Design review of the part built by this model. Coordinates are the model's own, in mm. Face numbers are marked on the shaded views. A direction names the side the tool comes from. Give positions to 0.01 mm unless a question says otherwise; leave off trailing zeros. Loops run counter-clockwise (first coordinate to the right, second up) from the corner with the lowest first, then second, coordinate; pieces in that order, holes last. Notation, with made-up numbers: (50, -19.5) - (77, -19.5) arc R35 ccw to (77, 12.5) - close; hole circle Ø9 at (45.5, -14). An arc over 180 degrees is marked (long way). One line per item, written item: value. Start each with the question number.
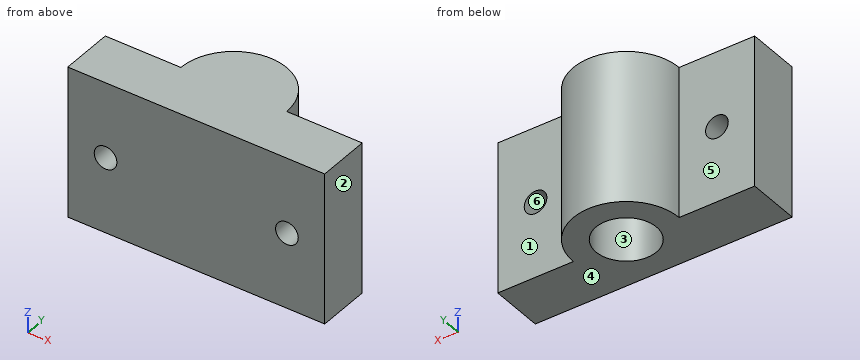
Autodesk Fusion 360 part; units mm, degrees
sketch "Sketch1" plane through (0, 0, 0) normal (0, 0, 1) x (1, 0, 0)
  circle A0 centre (0, 0) radius 4
  circle A1 centre (0, 0) radius 7
  line L0 (0, -6) -> (0, -7.3)
  line L1 (0, -7) -> (17, -7)
  line L2 (17, -7) -> (17, 0)
  line L3 (17, 0) -> (0, 0)
  line L4 (0, 0) -> (0, -7)
  line L5 (0, -7) -> (-17, -7)
  line L6 (-17, -7) -> (-17, 0)
  line L7 (-17, 0) -> (0, 0)
  line L8 (0, 0) -> (0, -7)
  line L9 (0.2459, 6.9957) -> (17, 0)
  line L10 (0.2459, 6.9957) -> (-17, 0)
  dimension "d1" = 8
  dimension "d2" = 14
  dimension "d3" = 17
  dimension "d4" = 7
extrude "Extrude1" add sketch "Sketch1" along normal blind 20 contours A0 A1 L0 L3 L4 L8 | A0 A1 L3 L7 L9 L10 | A0 A1 L0 L4 L7 L8 | A1 L1 L2 L3 | A1 L5 L6 L7 | A1 L9 | A1 L10
sketch "Sketch2" plane through (0, 0, 20) normal (0, 0, 1) x (-1, 0, 0)
  circle A0 centre (0, 0) radius 4
  line L0 (17, 7) -> (-17, 7)
  line L1 (-17, 7) -> (-17, 0)
  line L2 (-17, 0) -> (-7, 0)
  arc A1 (-7, 0) -> (7, 0) centre (0, 0) ccw
  line L3 (7, 0) -> (17, 0)
  line L4 (17, 0) -> (17, 7)
  circle A2 centre (0, 0) radius 4
extrude "Extrude2" add sketch "Sketch2" against normal blind 10 contours A0 A2
sketch "Sketch3" plane through (0, 0, 0) normal (0, 1, 0) x (-1, 0, 0)
  line L0 (-17, 0) -> (-7, 0)
  line L1 (-7, 0) -> (-7, 20)
  line L2 (-7, 20) -> (-17, 20)
  line L3 (-17, 20) -> (-17, 0)
  line L4 (-12, 0) -> (-12, 20) construction
  line L5 (-17, 10) -> (-7, 10) construction
  circle A0 centre (-12, 10) radius 1.5
  line L6 (0, 20) -> (0, 0) construction
  circle A1 centre (12, 10) radius 1.5
  dimension "d9" = 3
hole "Hole1" at (12, 0, 10) at (-12, 0, 10) direction (0, -1, 0) diameter 3 depth 11 tip angle 118
(1) Take a section at C-C on y = -5.5. State the section outline as (x, z) points, and give its area (3 significant figures).
(2) Draft analysis for pull direction Z (two halves, no side actions). For the marked faces 4, 5 and 6, state which applies: pulls with the +Z half, pulls with the -Z half, needs draft (parallel to the pull), parting line crosses it, or undercut.
(3) For pin 1 Ø11 at (x, z) = (-10.5, 13.5) entering from +Y; pin 2 Ø2 at (y, z) = (5.5, 8) entering from -X; pin 3 Ø5 at (x, z) = (12, 15) entering from +Y, all flat-tipped, find the tip position at first contact; note any pin that passes through.
(4) Take a section at A-A on z = 1.75. State the section outline as (x, y) points, and give its area (3 significant figures).
(5) Machinability: for the marked faces 1, 2 and 3, which of the approach directions +Z, -Z, +X, -X, +Y, -Y give a long, thin tool a straight path to every point of the face, cutting with its end or side? Answer none if there is none.
(6) Take a section at D-D on z = 16.75. State the section outline as (x, y) points, and give its area (3 significant figures).
(7) To check wall thickness, follow L1, parallel to X at y = -4.25, z = 10; L2, parallel to Z at x = -12, y = -5.25; L3, parallel to Y at x = -15.5, z = 11.5. State the ranges of each line that lie inside material, in increasing order. Write a range as from..to.
(8) Take a section at B-B on x = 12. State the section outline as (y, z) points.
Here are the results:
1. outline: (-17, 0) - (17, 0) - (17, 20) - (-17, 20) - close; hole circle Ø3 at (-12, 10); hole circle Ø3 at (12, 10)
1. area: 666 mm²
2. face 4: pulls with the -Z half
2. face 5: needs draft
2. face 6: undercut
3. pin 1: y = 4.9
3. pin 2: x = -5.36
3. pin 3: y = 0
4. outline: (-17, -7) - (17, -7) - (17, 0) - (7, 0) arc R7 ccw to (-7, 0) - (-17, 0) - close; hole circle Ø8 at (0, 0)
4. area: 265 mm²
5. face 1: +Z, -Z, +X, +Y
5. face 2: +Z, -Z, +X, +Y, -Y
5. face 3: -Z
6. outline: (-17, -7) - (17, -7) - (17, 0) - (7, 0) arc R7 ccw to (-7, 0) - (-17, 0) - close
6. area: 315 mm²
7. L1: -17..-13.5, -10.5..10.5, 13.5..17
7. L2: 0..8.5, 11.5..20
7. L3: -7..0
8. outline: (-7, 0) - (0, 0) - (0, 8.5) - (-7, 8.5) - close; (-7, 11.5) - (0, 11.5) - (0, 20) - (-7, 20) - close
